Check sheet for the modelled part. Datum: model origin and axes. Units: mm. A direction names the side the tool comes from. Round coordinates to 2 decimals unless told otherwise and drop trailing zeros. Write each loop counter-clockwise with the first axis right and the second up, starting at its lowest first coordinate (ties: lowest second). Pieces come first, ordered by that corner, then holes. Notation, with made-up numbers: M -10.75,65 L 29.25,65 A24 ccw 29.25,76 Z; hole C 47.25,-11 d7. An arc over 180 degrees is marked long. Put each result on its own line as item: value.
```python
from build123d import *

# Parameters (mm, degrees)
SKETCH1_W           = 140
SKETCH1_H           = 117.505
BOSS_EXTRUDE1_DEPTH = 6.35
SKETCH2_R           = 1.65
SKETCH2_R_2         = 7.5
SKETCH2_R_3         = 5.16
CUT_EXTRUDE1_DEPTH  = 7.35


with BuildPart() as part:
    # Sketch1 → Boss-Extrude1 (new body)
    with BuildSketch(Plane(origin=(0, 0, 0), x_dir=(1, 0, 0), z_dir=(0, 1, 0))):
        with Locations((70, 58.7525)):
            Rectangle(SKETCH1_W, SKETCH1_H)
    extrude(amount=BOSS_EXTRUDE1_DEPTH)

    # Sketch2 → Cut-Extrude1 (cut, through all)
    with BuildSketch(Plane(origin=(0, 6.35, 0), x_dir=(1, 0, 0), z_dir=(0, 1, 0))):
        with Locations((20, 10.675)):
            Circle(SKETCH2_R)
        with Locations((70, 64.265)):
            Circle(SKETCH2_R_2)
        with Locations((30.3125, 64.265)):
            Circle(SKETCH2_R_3)
        with Locations((120, 10.675)):
            Circle(SKETCH2_R)
        with Locations((109.6875, 64.265)):
            Circle(SKETCH2_R_3)
        with BuildLine():
            Line((18.35, 108.255), (18.35, 111.755))
            ThreePointArc((18.35, 111.755), (20, 113.405), (21.65, 111.755))
            Line((21.65, 111.755), (21.65, 108.255))
            ThreePointArc((21.65, 108.255), (20, 106.605), (18.35, 108.255))
        make_face()
        with BuildLine():
            Line((121.65, 108.255), (121.65, 111.755))
            ThreePointArc((121.65, 111.755), (120, 113.405), (118.35, 111.755))
            Line((118.35, 111.755), (118.35, 108.255))
            ThreePointArc((118.35, 108.255), (120, 106.605), (121.65, 108.255))
        make_face()
    extrude(amount=-CUT_EXTRUDE1_DEPTH, mode=Mode.SUBTRACT)


solid = part.part
```
1. Cross-section at B-B (x = 70). Enter the section's corners in (y, z) (3 decimals).
Computed values:
outline: M 0,-117.505 L 6.35,-117.505 L 6.35,-71.765 L 0,-71.765 Z; M 0,-56.765 L 6.35,-56.765 L 6.35,0 L 0,0 Z
2. Scan lines: probe 1 along X at (y, z) = (4.5, -111); probe 2 along X at (y, z) = (2.25, -10); probe 3 along Z at (x, y) = (66.5, 4.75) (3 decimals). Record each from-to range of solid material in increasing order.
Computed values:
probe 1: x = 0 to 18.35, 21.65 to 118.35, 121.65 to 140
probe 2: x = 0 to 18.49, 21.51 to 118.49, 121.51 to 140
probe 3: z = -117.505 to -70.898, -57.632 to 0
3. Cross-section at A-A (x = 120). Enter the section's corners in (y, z) (3 decimals).
Computed values:
outline: M 0,-117.505 L 6.35,-117.505 L 6.35,-113.405 L 0,-113.405 Z; M 0,-106.605 L 6.35,-106.605 L 6.35,-12.325 L 0,-12.325 Z; M 0,-9.025 L 6.35,-9.025 L 6.35,0 L 0,0 Z
4. Access from +Z, -Z, +X, -X, +Y, -Y to the whole of each face (thin tool, end or side, straight path). Record for faces 4 (the flat face through (69, 3, -117.505)), 5 (the cylindrical face through (119.964, 3.219, -106.605)).
Computed values:
face 4: -Z, +X, -X, +Y, -Y
face 5: +Y, -Y
5. Cross-section at C-C (y = 2). Count the separate pieces of the cut face and the enclosed holes in it, then the cut area to 3 significant figures.
Computed values:
separate pieces: 1
enclosed holes: 7
area: 16,000 mm2
6. Depth check by flat-ended pin: pin 1 Ø4 at (x, z) = (58.5, -20.5) entering from -Y. Enter the tip coordinate at first touch or a pass-through.
Computed values:
pin 1: stops at y = 0
7. Release check for a two-part mould opening along X. For faces 1 (the flat face through (140, 3, -58)), 2 (the flat face through (69, 0, -73)), 3 (the cylindrical face through (19.964, 3.219, -113.405)) record: +X half, -X half, draft (parallel to the pull), parting line (faces both ways), or undercut.
Computed values:
face 1: +X half
face 2: draft
face 3: undercut
